```python
from build123d import *

# Parameters (mm, degrees)
F0_W      = 193.0696666241
F0_H      = 200.0828683376
F1_DEPTH  = 214.122
F2_W      = 153.9536677301
F2_H      = 175.006001106
F3_DEPTH  = 25.4
F4_R      = 63.5
F5_DEPTH  = 150.368
F6_R      = 30.7008006584
F7_DEPTH  = 70.612
F7_TAPER  = -10
F9_DEPTH  = 366.776
F11_DEPTH = 193.0706666241


with BuildPart() as f1:
    # F0 (on Front) → F1 (new body)
    with BuildSketch(Plane.XZ):
        with Locations((-3.6960989237, -37.8023684025)):
            Rectangle(F0_W, F0_H)
    extrude(amount=F1_DEPTH)

    # F2 (on face) → F3 (join)
    with BuildSketch(Plane.XY.offset(62.2390657663)):
        with Locations((-3.6960989237, -107.061)):
            Rectangle(F2_W, F2_H)
    extrude(amount=F3_DEPTH)

    # F4 (on face) → F5 (cut)
    with BuildSketch(Plane.XY.offset(87.6390657663)):
        with Locations((-6.7443153821, -107.4839606881)):
            Circle(F4_R)
    extrude(amount=-F5_DEPTH, mode=Mode.SUBTRACT)

    # F6 (on face) → F7 (cut)
    with BuildSketch(Plane.XZ.offset(214.122)):
        with Locations((0, -9.5111001283)):
            Circle(F6_R)
    extrude(amount=-F7_DEPTH, taper=F7_TAPER, mode=Mode.SUBTRACT)

    # F8 (on face) → F9 (cut)
    with BuildSketch(Plane.YZ.offset(92.8387343884)):
        Polygon((-214.122, 62.2390657663), (-214.122, -10.3267068043), (-90.1689380407, 123.2789084315), (-194.4728940725, 123.2789084315), align=None)
    extrude(amount=-F9_DEPTH, mode=Mode.SUBTRACT)

    # F10 (on face) → F11 (cut, through all)
    with BuildSketch(Plane.YZ.offset(92.8387343884)):
        Polygon((-93.462087214, 101.8149778247), (0, -14.7983925417), (0, 62.2390657663), (-34.7359292209, 118.5938715935), align=None)
    extrude(amount=-F11_DEPTH, mode=Mode.SUBTRACT)


solid = f1.part
```
For this review, take the finished solid that the model builds, in its own axes (mm). A direction names the side the tool comes from. Give positions to 0.01 mm unless a question says otherwise; leave off trailing zeros. Write each loop counter-clockwise with the first axis right and the second up, starting at its lowest first coordinate (ties: lowest second). Pieces come first, ordered by that corner, then holes. Notation, with made-up numbers: M -2,-20 L 3,-20 A22 ccw 3,-5 Z; hole C 74,77.5 d7. An arc over 180 degrees is marked long. Answer as CSV lines item,"result".
1. Consider section D-D, the plane x = 0. Write out the cut boundary in (y, z).
Findings:
outline,"M -214.12,-137.84 L 0,-137.84 L 0,-14.8 L -44.34,40.53 L -44.34,-62.73 L -170.62,-62.73 L -170.62,-47.88 L -214.12,-40.21 Z; M -179.16,27.35 L -170.62,28.86 L -170.62,36.56 Z"
2. For pin 1 (6 mm diameter, centred on x = -93, y = -94.5, fed in from +Z); pin 2 (6 mm diameter, centred on x = 64.5, y = -30.5, fed in from +Z), all flat-tipped, find the tip position at first contact; note any pin that passes through.
Findings:
pin 1,"stops at z = 62.24"
pin 2,"stops at z = 27"
3. For faces 5 (the flat face through (-91, -104, 62.239)), 6 (the conical face through (16.31, -187.82, -40.86)), 7 (the flat face through (83, -104, 62.239)), 8 (the cylindrical face through (-15.011, -44.524, -3.2)), list the 3-axis set-ups (+Z, -Z, +X, -X, +Y, -Y) from which the entire face can be reached by the end or side of a thin tool; tool diameter is ignored.
Findings:
face 5,"+Z, -X, +Y, -Y"
face 6,"none"
face 7,"+Z, +X, +Y, -Y"
face 8,"+Z"
4. Wall thickness on line 1 (X direction, y = -108, z = 26.5); line 2 (Z direction, x = -68, y = -35); line 3 (Y direction, x = -42, z = 6.5): over which ranges is each line inside the solid? List them lowest first.
Findings:
line 1,"x = -100.23 to -70.24, 56.75 to 92.84"
line 2,"z = -137.84 to 28.87"
line 3,"y = -198.51 to -160.3, -54.67 to -17.07"
5. Consider section C-C, the plane z = 68. Write out the cut boundary in (x, y).
Findings:
outline,"M -80.67,-141.45 L -60.39,-141.45 A63.5 cw -55.13,-66.36 L -80.67,-66.36 Z; M 41.64,-66.36 A63.5 cw 46.91,-141.45 L 73.28,-141.45 L 73.28,-66.36 Z"
6. Consider section B-B, the plane y = -178. Write out the cut boundary in (x, z), then the cut area to 3 significant figures.
Findings:
outline,"M -100.23,-137.84 L 92.84,-137.84 L 92.84,28.61 L -100.23,28.61 Z; hole C 0,-9.51 d74.14"
area,"27,800 mm2"
7. Consider section A-A, the plane x = 61. Write out the cut boundary in (y, z), then the cut area to 3 significant figures.
Findings:
outline,"M -214.12,-137.84 L 0,-137.84 L 0,-14.8 L -82.1,87.64 L -123.23,87.64 L -214.12,-10.33 Z"
area,"39,600 mm2"
8. Draft analysis for pull direction X (two halves, no side actions). For faces 1 (the flat face through (-75, -102, 87.639)), 2 (the flat face through (-80.673, -105, 72)), 3 (the flat face through (73.281, -105, 72)), 4 (the flat face through (-8, -107, -62.729)), state which applies: +X half, -X half, draft (parallel to the pull), parting line (faces both ways), or undercut.
Findings:
face 1,"draft"
face 2,"-X half"
face 3,"+X half"
face 4,"undercut"
